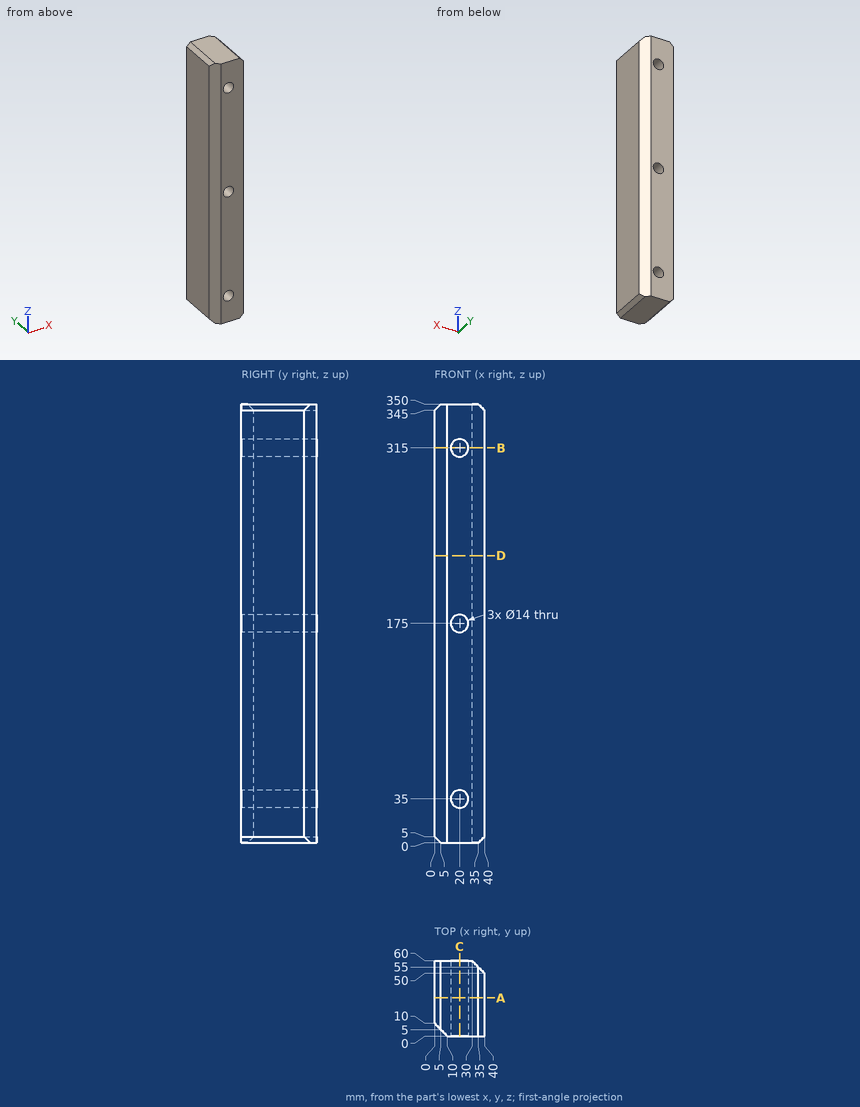
The figure shows three views and two pictorial views of one solid part (mm, origin at its lowest corner). Answer the questions. Give positions to 0.01 mm unless a question says otherwise; leave off trailing zeros. Write each loop counter-clockwise with the first axis right and the second up, starting at its lowest first coordinate (ties: lowest second). Pieces come first, ordered by that corner, then holes. Notation, with made-up numbers: (22.5, 58.25) - (30.5, 58.25) arc R10 ccw to (30.5, 68.25) - close; hole circle Ø1 at (18, 86). An arc over 180 degrees is marked (long way). Use one line per item in the form item = value.
1. A cutting plane is placed at C-C (x = 20). Write down the section's boundary in (y, z), and give its area (3 significant figures).
Filled in:
outline = (0, 0) - (60, 0) - (60, 28) - (0, 28) - close; (0, 42) - (60, 42) - (60, 168) - (0, 168) - close; (0, 182) - (60, 182) - (60, 308) - (0, 308) - close; (0, 322) - (60, 322) - (60, 350) - (0, 350) - close
area = 18,500 mm^2
2. Consider L1, parallel to Z at x = 21, y = 35.5; L2, parallel to Z at x = 16, y = 13.5; L3, parallel to X at y = 21, z = 175. Determine where each line is inside the solid, lowest interval first.
Filled in:
L1 = 0 to 28.07, 41.93 to 168.07, 181.93 to 308.07, 321.93 to 350
L2 = 0 to 29.26, 40.74 to 169.26, 180.74 to 309.26, 320.74 to 350
L3 = 0 to 13, 27 to 40
3. A cutting plane is placed at D-D (z = 229). Write down the section's boundary in (x, y).
Filled in:
outline = (0, 10) - (10, 0) - (40, 0) - (40, 50) - (30, 60) - (0, 60) - close
4. A cutting plane is placed at A-A (y = 30.5). Write down the section's boundary in (x, z), and give its area (3 significant figures).
Filled in:
outline = (0, 5) - (5, 0) - (35, 0) - (40, 5) - (40, 345) - (35, 350) - (5, 350) - (0, 345) - close; hole circle Ø14 at (20, 35); hole circle Ø14 at (20, 175); hole circle Ø14 at (20, 315)
area = 13,500 mm^2
5. A cutting plane is placed at B-B (z = 315). Write down the section's boundary in (x, y), and give its area (3 significant figures).
Filled in:
outline = (0, 10) - (10, 0) - (13, 0) - (13, 60) - (0, 60) - close; (27, 0) - (40, 0) - (40, 50) - (30, 60) - (27, 60) - close
area = 1,460 mm^2
